Input: part model. Units: mm. Frame: model coordinates. A direction names the side the tool comes from. Round coordinates to 2 decimals unless told otherwise and drop trailing zeros. Loops run counter-clockwise (first coordinate to the right, second up) from the corner with the lowest first, then second, coordinate; pieces in that order, holes last.
1) Section A-A, the plane x = 7.75. Return loops of the section in (y, z), and give its area (3 significant figures).
2) Section C-C, the plane x = 6.35. Return loops of the section in (y, z), and give its area (3 significant figures).
3) Access query for faces 4 (the face through (2.53, 3.86, 16.25)), 5 (the face through (0, 4, 6)). Directions: +Z, -Z, +X, -X, +Y, -Y. A direction counts if a zero-diameter tool reaches every point of the face in a straight line with its end or side. Return the directions, or none.
4) Section B-B, the plane y = 6. Return loops of the section in (x, z), and give its area (3 significant figures).
5) First-contact query: pin 1 (2 mm diameter, centred on x = 1.5, z = 14.5, fed in from +Y). Flat tip, straight axial feed; report the tip coordinate or a pass-through.
6) Draft query along X for faces 1 (the face through (7.93, 3.86, 16.18)), 2 (the face through (9.355, 3.863, 15.654)), 3 (the face through (8, 4, 18.872)). Return one class per face: pulls with the +X half, pulls with the -X half, needs draft (parallel to the pull), parting line crosses it, or undercut.
7) Section D-D, the plane y = 8.25. Return loops of the section in (x, z).
8) Ray query, line 1 along Y through (x, z) = (4.25, 4.5); line 2 along X through (y, z) = (7.25, 14); line 3 along X through (y, z) = (2.25, 14.25). Return the intervals inside material, ascending.
from build123d import *

# Parameters (mm, degrees)
HFBR_BASE_W          = 10.2
HFBR_BASE_H          = 12.3444
EXTRUDE1_DEPTH       = 7.62
EXTRUDE2_DEPTH       = 7.62
SKETCH3_R            = 0.254
PINS_DEPTH           = 3.81
LPATTERN1_COUNT      = 4
LPATTERN1_PITCH      = 2.54
LPATTERN1_COUNT_DIR2 = 2
LPATTERN1_PITCH_DIR2 = 7.62


with BuildPart() as part:
    # HFBR Base → Extrude1 (new body)
    with BuildSketch(Plane(origin=(0, 0, 0), x_dir=(1, 0, 0), z_dir=(0, 1, 0))):
        with Locations((5.1, -6.1722)):
            Rectangle(HFBR_BASE_W, HFBR_BASE_H)
    extrude(amount=EXTRUDE1_DEPTH)

    # Sketch2 → Extrude2 (add)
    with BuildSketch(Plane(origin=(0, 7.62, 0), x_dir=(-1, 0, 0), z_dir=(0, 1, 0))):
        Polygon((0, 12.3444), (-2.056727008, 18.8722), (-3.326727008, 18.8722), (-1.71375929, 13.55750012), (-8.579624915, 13.55750012), (-7.263727008, 18.8722), (-8.533727008, 18.8722), (-10.2, 12.3444), align=None)
    extrude(amount=-EXTRUDE2_DEPTH)

    # Sketch3 → Pins (add)
    with BuildSketch(Plane(origin=(0, 7.62, 0), x_dir=(-1, 0, 0), z_dir=(0, 1, 0))):
        with Locations((-1.27, 2.9972)):
            Circle(SKETCH3_R)
    pins = extrude(amount=PINS_DEPTH)

    # LPattern1: Pins 4 × 2, 2 skipped
    with Locations(*[(i * LPATTERN1_PITCH, 0, j * LPATTERN1_PITCH_DIR2) for i in range(LPATTERN1_COUNT) for j in range(LPATTERN1_COUNT_DIR2) if (i, j) not in ((0, 0), (1, 1), (2, 1))]):
        add(pins)


solid = part.part
Final values:
1. outline: (0, 0) - (7.62, 0) - (7.62, 13.56) - (0, 13.56) - close; (0, 16.91) - (7.62, 16.91) - (7.62, 18.87) - (0, 18.87) - close
1. area: 118 mm2
2. outline: (0, 0) - (7.62, 0) - (7.62, 2.74) - (11.43, 2.74) - (11.43, 3.25) - (7.62, 3.25) - (7.62, 13.56) - (0, 13.56) - close
2. area: 105 mm2
3. face 4: +Y, -Y
3. face 5: +Z, -Z, -X, +Y, -Y
4. outline: (0, 0) - (10.2, 0) - (10.2, 12.34) - (8.53, 18.87) - (7.26, 18.87) - (8.58, 13.56) - (1.71, 13.56) - (3.33, 18.87) - (2.06, 18.87) - (0, 12.34) - close
4. area: 152 mm2
5. pin 1: stops at y = 7.62
6. face 1: undercut
6. face 2: pulls with the +X half
6. face 3: needs draft
7. outline: circle Ø0.51 at (1.27, 3); circle Ø0.51 at (1.27, 10.62); circle Ø0.51 at (3.81, 3); circle Ø0.51 at (6.35, 3); circle Ø0.51 at (8.89, 3); circle Ø0.51 at (8.89, 10.62)
8. line 1: y = 0 to 7.62
8. line 2: x = 0.52 to 1.85, 8.47 to 9.78
8. line 3: x = 0.6 to 1.92, 8.41 to 9.71
